from build123d import *

# Parameters (mm, degrees)
SKETCH2_W       = 10.5156
SKETCH2_H       = 1.905
SLOT_DEPTH      = 2.7686
HOLE_DEPTH      = 27.149259908
HOLE_DEPTH_BACK = 27.149259908
SKETCH5_R       = 0.7874
THDSCHPAT_COUNT = 15
THDSCHPAT_PITCH = 1.27


with BuildPart() as part:
    # BodySke → Base-Revolve (revolve)
    with BuildSketch(Plane.XY, mode=Mode.PRIVATE) as base_revolve_sk:
        with BuildLine():
            Line((6.0198, 3.175), (6.0198, 5.2578))
            Line((6.0198, 5.2578), (1.7018, 5.2578))
            ThreePointArc((1.7018, 5.2578), (0.436044816, 2.763176799), (0, 0))
            Line((0, 0), (25.0698, 0))
            Line((25.0698, 0), (25.0698, 3.175))
            Line((25.0698, 3.175), (6.0198, 3.175))
        make_face()
    revolve(base_revolve_sk.sketch.rotate(Axis((-25.4, 0, 0), (1, 0, 0)), 90), axis=Axis((-25.4, 0, 0), (1, 0, 0)))

    # Sketch2 → Slot (cut)
    with BuildSketch(Plane(origin=(0, 0, 0), x_dir=(0, 0, -1), z_dir=(1, 0, 0))):
        Rectangle(SKETCH2_W, SKETCH2_H)
    extrude(amount=SLOT_DEPTH, mode=Mode.SUBTRACT)

    # Sketch5 → Hole (cut, two sides: drawn at the far end of the back side and taken through both)
    with BuildSketch(Plane(origin=(0, 0, 0), x_dir=(1, 0, 0), z_dir=(0, 1, 0)).offset(-HOLE_DEPTH_BACK)):
        with Locations(Location((4.445, 0, 0), (0, 0, 270))):
            Circle(SKETCH5_R)
    extrude(amount=HOLE_DEPTH + HOLE_DEPTH_BACK, mode=Mode.SUBTRACT)

    # ThdSchSke → ThreadSchematic (revolve, cut)
    with BuildSketch(Plane.XY):
        Polygon((7.2898, -2.41935), (6.760688174, -3.175), (6.760688174, -3.96875), (7.818911826, -3.96875), (7.818911826, -3.175), align=None)
    threadschematic = revolve(axis=Axis((-3.175, 0, 0), (1, 0, 0)), mode=Mode.SUBTRACT)

    # ThdSchPat: ThreadSchematic ×15
    with Locations(*[(i * THDSCHPAT_PITCH, 0, 0) for i in range(1, THDSCHPAT_COUNT)]):
        add(threadschematic, mode=Mode.SUBTRACT)


solid = part.part
Geometry: final body of the model. Coordinates: model frame, mm. Give positions to 0.01 mm unless a question says otherwise; leave off trailing zeros. Loops run counter-clockwise (first coordinate to the right, second up) from the corner with the lowest first, then second, coordinate; pieces in that order, holes last. Notation, with made-up numbers: M 75.25,-7.5 L 106.25,-7.5 A21 cw 106.25,16.5 Z; hole C 52,83 d1. An arc over 180 degrees is marked long. Put each result on its own line as item: value. Start each with the question number.
1) Cut plane C-C (y = -2.75). Give the number of separate pieces and of enclosed holes in the cut face, then the cut area to 3 significant figures.
2) Cut plane B-B (y = 4). Output: boundary loops of the cut face in (x, z) (3 decimals), then the cut area to 3 significant figures.
3) Pull-direction query (Z, two-part tool) for faces 1 (the cylindrical face through (6.39, -0.95, 3.03)), 2 (the cylindrical face through (5.226, -0.074, -0.103)), 3 (the flat face through (2, -0.952, 0)); classes: pulls with the +Z half, pulls with the -Z half, needs draft (parallel to the pull), parting line crosses it, or undercut.
4) Contact query for flat-ended pins moving along their axis: pin 1 (2 mm diameter, centred on y = -4, z = 3, fed in from +X); pin 2 (2 mm diameter, centred on x = 6, y = -2.5, fed in from +Z); pin 3 (2 mm diameter, centred on x = 1, z = -2, fed in from -Y). Output: stop coordinate, or through.
5) Cut plane A-A (x = 2.25). Output: boundary loops of the cut face in (y, z), then the cut area to 3 significant figures.
6) Ray query, line 1 along X through (y, z) = (-0.25, 2); line 2 along X through (y, z) = (1.5, 0); line 3 along Y through (x, z) = (2.5, 3.25). Return the intervals inside material, ascending.
Verdict:
1. separate pieces: 15
1. enclosed holes: 1
1. area: 74.2 mm2
2. outline: M 1.702,-3.412 L 6.02,-3.412 L 6.02,3.412 L 1.702,3.412 A8.032 ccw Z; hole C 4.445,0 d1.575
2. area: 31.0 mm2
3. face 1: parting line crosses it
3. face 2: undercut
3. face 3: needs draft
4. pin 1: x = 6.02
4. pin 2: z = 5.04
4. pin 3: y = -5.1
5. outline: M -0.95,-5.17 L -0.95,5.17 A5.26 ccw Z; M 0.95,-5.17 A5.26 ccw 0.95,5.17 Z
5. area: 66.9 mm2
6. line 1: 2.77 to 25.07
6. line 2: 0.13 to 3.66, 5.23 to 25.07
6. line 3: -4.13 to -0.95, 0.95 to 4.13
